```python
from build123d import *

# Parameters (mm, degrees)
SKETCH1_R           = 3.375
BOSS_EXTRUDE1_DEPTH = 1.65
SKETCH2_R           = 1.5
BOSS_EXTRUDE2_DEPTH = 10.35
CHAMFER1_SIZE       = 0.3
CUT_EXTRUDE1_DEPTH  = 2
CHAMFER2_SIZE       = 1.65


with BuildPart() as part:
    # Sketch1 → Boss-Extrude1 (new body)
    with BuildSketch(Plane.XY):
        Circle(SKETCH1_R)
    extrude(amount=BOSS_EXTRUDE1_DEPTH)

    # Sketch2 → Boss-Extrude2 (add)
    with BuildSketch(Plane(origin=(0, 0, 0), x_dir=(-1, 0, 0), z_dir=(0, 0, -1))):
        with Locations(Location((0, 0, 0), (0, 0, 180))):
            Circle(SKETCH2_R)
    extrude(amount=BOSS_EXTRUDE2_DEPTH)

    # Chamfer1
    chamfer1_edges = [part.edges().sort_by_distance(p)[0] for p in [
        (-1.5, 0, -10.35),
    ]]
    chamfer(chamfer1_edges, length=CHAMFER1_SIZE)

    # Sketch3 → Cut-Extrude1 (cut)
    with BuildSketch(Plane.XY.offset(1.65)):
        Polygon((0, 1.154700538), (-1, 0.577350269), (-1, -0.577350269), (0, -1.154700538), (1, -0.577350269), (1, 0.577350269), align=None)
    extrude(amount=-CUT_EXTRUDE1_DEPTH, mode=Mode.SUBTRACT)

    # Chamfer2
    chamfer2_edges = [part.edges().sort_by_distance(p)[0] for p in [
        (-3.375, 0, 0),
    ]]
    chamfer(chamfer2_edges, length=CHAMFER2_SIZE - 0.0001)  # a hair under: the kernel refuses the full size


solid = part.part
```
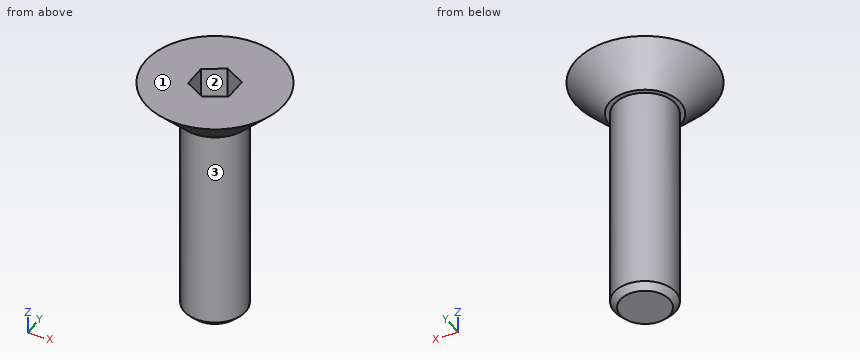
For this review, take the finished solid that the model builds, in its own axes (mm). Face numbers are marked on the shaded views. A direction names the side the tool comes from. Round coordinates to 2 decimals unless told otherwise and drop trailing zeros. Order: outer loops, then holes, each group sorted by start corner. A loop starts at its lowest first (then second) coordinate and runs counter-clockwise, first axis right, second up.
Q1. Machinability: for the marked faces 1, 2 and 3, which of the approach directions +Z, -Z, +X, -X, +Y, -Y give a long, thin tool a straight path to every point of the face, cutting with its end or side? Answer none if there is none.
Findings below:
face 1: +Z, +X, -X, +Y, -Y
face 2: +Z
face 3: -Z
Q2. Insertion check: P1, Ø4, axis at x = 0.5, z = -5.5, coming from the +Y side; P2, Ø0.6, axis at y = 0, z = 0.5, coming from the +X side; P3, Ø2, axis at y = 1, z = -6.5, coming from the -X side. Each pin has a flat end and moves straight along its axis. Give the tip position at first contact, or say it passes through.
Findings below:
P1: stops at y = 1.5
P2: stops at x = 2.53
P3: stops at x = -1.5
Q3. Wall thickness on line 1 (Z direction, x = 1.5, y = 1.75); line 2 (X direction, y = -1.25, z = -4.5); line 3 (X direction, y = 1, z = -1.75): over which ranges is each line inside the solid? List them lowest first.
Findings below:
line 1: z = 0.58 to 1.65
line 2: x = -0.83 to 0.83
line 3: x = -1.12 to 1.12
Q4. We need section B-B, the plane z = -9.5. Give the boundary of the cut face in (x, y).
Findings below:
outline: circle Ø3 at (0, 0)
